Build history of the part. All positions in model axes, mm. Face numbers are marked on the shaded views. A direction names the side the tool comes from. Round coordinates to 2 decimals unless told otherwise and drop trailing zeros. Write each loop counter-clockwise with the first axis right and the second up, starting at its lowest first coordinate (ties: lowest second). Pieces come first, ordered by that corner, then holes.
1) Saw through at B-B (z = 2.5). State how many separate pieces and enclosed holes the cut face has, plus the area to 3 significant figures.
2) Wall check: probe 1 along Y at (x, z) = (0, 0.7); probe 2 along Z at (x, y) = (-10, 20.5); probe 3 along X at (y, z) = (1.5, 2.5). Give the ranges that are in metal, low to high.
3) Saw through at C-C (y = 20.5). Write the cut outline in (x, z).
4) Flat gauge pins, fed straight in: pin 1 (0.6 mm diameter, centred on y = 30.5, z = 3, fed in from +X); pin 2 (1.1 mm diameter, centred on y = 29, z = 1.5, fed in from -X); pin 3 (5 mm diameter, centred on x = -4, z = 4, fed in from -Y); pin 4 (2.5 mm diameter, centred on x = 0, y = 30.5, fed in from +Z). Where does each tip first touch, or does it go through?
5) Which spindle directions (+Z, -Z, +X, -X, +Y, -Y) get a long thin tool onto all of the face, cutting with end or side? Do the marked faces 4, 5 and 6. Say none if no direction does.
6) Saw through at D-D (y = 1). Write the cut outline in (x, z), plus the area to 3 significant figures.
7) Pull direction Y, two halves, no side cores. Call the marked faces 1, 2 and 3: +Y half, -Y half, draft (parallel to the pull), parting line (faces both ways), or undercut.
8) Saw through at A-A (x = -10). Write the cut outline in (y, z).
from build123d import *

# Parameters (mm, degrees)
F0_R      = 1.6
F1_DEPTH  = 4
F2_W      = 35
F2_H      = 12
F3_DEPTH  = 6
F4_R      = 1.6
F5_DEPTH  = 20.751
F6_R      = 0.8
F7_R      = 1.5
F8_DEPTH  = 35.001
F10_DEPTH = 2.2
F11_R     = 0.2


with BuildPart() as f1:
    # F0 (on Top) → F1 (new body)
    with BuildSketch(Plane.XY):
        with BuildLine():
            ThreePointArc((5, 30.25), (0, 35.25), (-5, 30.25))
            Line((-5, 30.25), (-5, 26.5))
            Line((-5, 26.5), (-17.5, 26.5))
            Line((-17.5, 26.5), (-17.5, 14.5))
            Line((-17.5, 14.5), (-5, 14.5))
            Line((-5, 14.5), (-5, 0))
            ThreePointArc((-5, 0), (0, -5), (5, 0))
            Line((5, 0), (5, 14.5))
            Line((5, 14.5), (17.5, 14.5))
            Line((17.5, 14.5), (17.5, 26.5))
            Line((17.5, 26.5), (5, 26.5))
            Line((5, 26.5), (5, 30.25))
        make_face()
        Circle(F0_R, mode=Mode.SUBTRACT)
        with Locations((0, 30.25)):
            Circle(F0_R, mode=Mode.SUBTRACT)
    extrude(amount=F1_DEPTH)

    # F2 (on face) → F3 (join)
    with BuildSketch(Plane.XY.offset(4)):
        with Locations((0, 20.5)):
            Rectangle(F2_W, F2_H)
    extrude(amount=F3_DEPTH)

    # F4 (on face) → F5 (cut, through all)
    with BuildSketch(Plane.XZ.offset(-14.5)):
        with Locations((-10, 7.5)):
            Circle(F4_R)
        with Locations((10, 7.5)):
            Circle(F4_R)
    extrude(amount=-F5_DEPTH, mode=Mode.SUBTRACT)

    # F6
    f6_edges = [f1.edges().sort_by_distance(p)[0] for p in [
        (0, 26.5, 10),
        (-17.5, 20.5, 10),
        (0, 14.5, 10),
        (17.5, 20.5, 10),
    ]]
    fillet(f6_edges, radius=F6_R)

    # F7 (on face) → F8 (cut, through all)
    with BuildSketch(Plane.YZ.offset(17.5)):
        with Locations((20.5, 2.5)):
            Circle(F7_R)
    extrude(amount=-F8_DEPTH, mode=Mode.SUBTRACT)

    # F9 (on face) → F10 (cut)
    with BuildSketch(Plane.XY.offset(4)):
        Polygon((-2.6846787517, 28.7), (0, 27.15), (2.6846787517, 28.7), (2.6846787517, 31.8), (0, 33.35), (-2.6846787517, 31.8), align=None)
        Polygon((2.6846787517, 1.55), (0, 3.1), (-2.6846787517, 1.55), (-2.6846787517, -1.55), (0, -3.1), (2.6846787517, -1.55), align=None)
    extrude(amount=-F10_DEPTH, mode=Mode.SUBTRACT)

    # F11
    f11_edges = [f1.edges().sort_by_distance(p)[0] for p in [
        (5, 7.25, 4),
        (0, -5, 4),
        (0, 14.5, 4),
        (-5, 7.25, 4),
        (2.684679, 0, 4),
        (1.342339, 2.325, 4),
        (-1.342339, 2.325, 4),
        (-2.684679, 0, 4),
        (-1.342339, -2.325, 4),
        (1.342339, -2.325, 4),
        (5, 28.375, 4),
        (0, 26.5, 4),
        (0, 35.25, 4),
        (-5, 28.375, 4),
        (-1.342339, 27.925, 4),
        (1.342339, 27.925, 4),
        (2.684679, 30.25, 4),
        (1.342339, 32.575, 4),
        (-1.342339, 32.575, 4),
        (-2.684679, 30.25, 4),
        (-5, 30.25, 2),
        (-5, 26.5, 2),
        (-5, 28.375, 0),
        (11.25, 26.5, 0),
        (5, 26.5, 2),
        (-11.25, 26.5, 0),
        (0, 35.25, 0),
        (5, 28.375, 0),
        (-5, 14.5, 2),
        (5, 14.5, 2),
    ]]
    fillet(f11_edges, radius=F11_R)


solid = f1.part
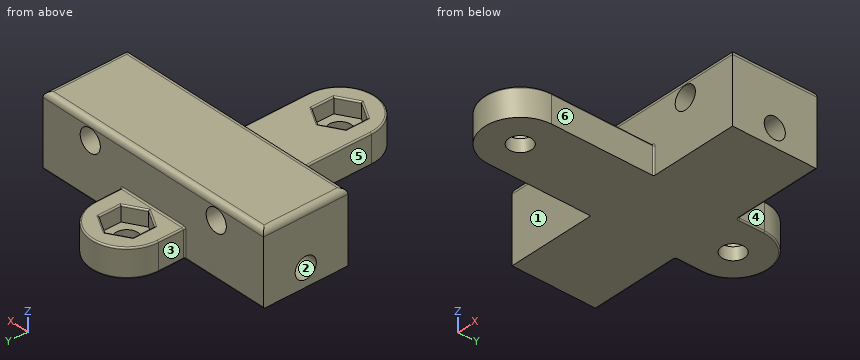
Evaluation:
1. separate pieces: 2
1. enclosed holes: 2
1. area: 526 mm2
2. probe 1: y = -5 to -1.6, 1.6 to 28.65, 31.85 to 35.25
2. probe 2: z = 0 to 1, 4 to 5.9, 9.1 to 10
2. probe 3: x = -5 to -2.68, 2.68 to 5
3. outline: (-17.5, 0) - (17.5, 0) - (17.5, 1) - (-17.5, 1) - close; (-17.5, 4) - (17.5, 4) - (17.5, 9.2) arc R0.8 ccw to (16.7, 10) - (-16.7, 10) arc R0.8 ccw to (-17.5, 9.2) - close; hole circle Ø3.2 at (-10, 7.5); hole circle Ø3.2 at (10, 7.5)
4. pin 1: stops at x = 5
4. pin 2: stops at x = -5
4. pin 3: stops at y = -4.77
4. pin 4: passes through
5. face 4: +Z, -Z, +X, +Y
5. face 5: +Z, -Z, -X, -Y
5. face 6: +Z, -Z, +X, -Y
6. outline: (-5, 0) - (-1.25, 0) - (-1.25, 1.8) - (-2.68, 1.8) - (-2.68, 3.8) arc R0.2 ccw to (-2.88, 4) - (-4.8, 4) arc R0.2 ccw to (-5, 3.8) - close; (1.25, 0) - (5, 0) - (5, 3.8) arc R0.2 ccw to (4.8, 4) - (2.88, 4) arc R0.2 ccw to (2.68, 3.8) - (2.68, 1.8) - (1.25, 1.8) - close
6. area: 23.7 mm2
7. face 1: -Y half
7. face 2: undercut
7. face 3: draft
8. outline: (14.5, 0) - (26.3, 0) arc R0.2 ccw to (26.5, 0.2) - (26.5, 5.9) - (14.5, 5.9) - close; (14.5, 9.1) - (26.5, 9.1) - (26.5, 9.2) arc R0.8 ccw to (25.7, 10) - (15.3, 10) arc R0.8 ccw to (14.5, 9.2) - close; hole circle Ø3 at (20.5, 2.5)
